Here's how the part is built. I have some questions about the finished solid (model axes, mm). A direction names the side the tool comes from. Give positions to 0.01 mm unless a question says otherwise; leave off trailing zeros. Loops run counter-clockwise (first coordinate to the right, second up) from the corner with the lowest first, then second, coordinate; pieces in that order, holes last. Notation, with made-up numbers: (-35.5, 56.5) - (-27.5, 56.5) arc R23 ccw to (-27.5, 90.5) - close; hole circle Ø5 at (83, 32). An arc over 180 degrees is marked (long way). Return JSON: item names as keys, results as strings. Group by question number.
(1) If we section it at D-D (z = 17.75): Please give me the cut outline in (x, y).
(2) If we mould it in two halves opening along X, with no side actions, what happens to faces 1 (the flat face through (-7.5, 26, 11)), 2 (the flat face through (41, 5, 14.45)), 3 (the flat face through (42.8, 5, 17))? For each: released by +X, released by -X, zero draft, split by the parting line, or undercut.
(3) If we section it at C-C (z = 10.5): Please give me the cut outline in (x, y).
(4) If we section it at B-B (y = 8): Please give me the cut outline in (x, z).
(5) On a 3-axis mill with a long thin cutter (end or side, diameter ignored), from which of +Z, -Z, +X, -X, +Y, -Y can I reach the whole of each face in a straight line? I mean faces 4 (the flat face through (28, 5, 2.5)), 5 (the flat face through (28, -90, 5)), 6 (the flat face through (-4, 26, 2.5)). Say none if no direction works.
(6) If we section it at A-A (x = 16.5): Please give me the cut outline in (y, z), then the cut area to 3 significant figures.
(7) For P1, Ø1, axis at y = -84, z = 10, coming from the +X side; P2, Ø0.7, axis at x = 7, z = 9, coming from the -Y side; P3, Ø8, axis at x = 25.5, y = 5, coming from the -Z side; P4, Ø2, axis at x = 30, z = 12.5, coming from the -Y side, each with a flat end and sliding along its axis, tell me the tip position at first contact or that it passes through.
(8) I need wall thicknesses on probe 1 along Y at (x, z) = (32, 6.25); probe 2 along X at (y, z) = (-111, 16); probe 3 along X at (y, z) = (8, 6). Which ranges of each line are inside material? Lowest first, please. Write a range as [from, to].
```python
from build123d import *

# Parameters (mm, degrees)
BOSS_EXTRUDE1_DEPTH      = 21.9
SKETCH2_W                = 4.7
SKETCH2_H                = 10
BOSS_EXTRUDE2_DEPTH      = 30
SKETCH3_W                = 5
SKETCH3_H                = 21.9
BOSS_EXTRUDE3_DEPTH      = 120
SKETCH4_W                = 3
SKETCH4_H                = 10
BOSS_EXTRUDE4_DEPTH      = 0.25
SKETCH5_W                = 3
SKETCH5_H                = 10
BOSS_EXTRUDE5_DEPTH      = 0.25
CORTE_EXTRUS_O1_DEPTH    = 10
ESBO_O3_W                = 21.9
ESBO_O3_H                = 7.5
RESSALTO_EXTRUS_O2_DEPTH = 10
ESBO_O4_W                = 7.5
ESBO_O4_H                = 16.9
CORTE_EXTRUS_O2_DEPTH    = 10
PADR_O_LINEAR1_COUNT     = 2
PADR_O_LINEAR1_PITCH     = 100


with BuildPart() as part:
    # Sketch1 → Boss-Extrude1 (new body)
    with BuildSketch(Plane.XY):
        Polygon((0, 0), (0, 30), (12.8, 30), (12.8, 0), (7.8, 0), (7.8, 10), (6, 10), (6, 0), align=None)
    extrude(amount=BOSS_EXTRUDE1_DEPTH)

    # Sketch2 → Boss-Extrude2 (add)
    with BuildSketch(Plane(origin=(12.8, 0, 0), x_dir=(0, 0, -1), z_dir=(1, 0, 0))):
        with Locations((-17.05, 5)):
            Rectangle(SKETCH2_W, SKETCH2_H)
        with Locations((-4.85, 5)):
            Rectangle(SKETCH2_W, SKETCH2_H)
    boss_extrude2 = extrude(amount=BOSS_EXTRUDE2_DEPTH)

    # Sketch3 → Boss-Extrude3 (add)
    with BuildSketch(Plane.XZ):
        with Locations((10.3, 10.95)):
            Rectangle(SKETCH3_W, SKETCH3_H)
    extrude(amount=BOSS_EXTRUDE3_DEPTH)

    # Sketch4 → Boss-Extrude4 (add)
    with BuildSketch(Plane(origin=(0, 0, 14.7), x_dir=(-1, 0, 0), z_dir=(0, 0, -1))):
        with Locations((-41.3, 5)):
            Rectangle(SKETCH4_W, SKETCH4_H)
    boss_extrude4 = extrude(amount=BOSS_EXTRUDE4_DEPTH)

    # Sketch5 → Boss-Extrude5 (add)
    with BuildSketch(Plane.XY.offset(7.2)):
        with Locations((41.3, 5)):
            Rectangle(SKETCH5_W, SKETCH5_H)
    boss_extrude5 = extrude(amount=BOSS_EXTRUDE5_DEPTH)

    # Esboço2 → Corte-extrusão1 (cut)
    with BuildSketch(Plane.XZ):
        with BuildLine():
            Line((6, 21.9), (6, 0))
            ThreePointArc((6, 0), (5.377380148, 10.95), (6, 21.9))
        make_face()
    extrude(amount=-CORTE_EXTRUS_O1_DEPTH, mode=Mode.SUBTRACT)

    # Esboço3 → Ressalto-extrusão2 (add)
    with BuildSketch(Plane.ZY):
        with Locations((10.95, 26.25)):
            Rectangle(ESBO_O3_W, ESBO_O3_H)
    extrude(amount=RESSALTO_EXTRUS_O2_DEPTH)

    # Esboço4 → Corte-extrusão2 (cut)
    with BuildSketch(Plane.XZ.offset(-22.5)):
        with Locations((-3.75, 10.95)):
            Rectangle(ESBO_O4_W, ESBO_O4_H)
    extrude(amount=-CORTE_EXTRUS_O2_DEPTH, mode=Mode.SUBTRACT)

    # Padrão linear1: Boss-Extrude2, Boss-Extrude4, Boss-Extrude5 ×2
    with Locations(*[(0, -i * PADR_O_LINEAR1_PITCH, 0) for i in range(1, PADR_O_LINEAR1_COUNT)]):
        add(boss_extrude2)
        add(boss_extrude4)
        add(boss_extrude5)


solid = part.part
```
Values:
{
 "1": {"outline": "(-10, 22.5) - (-7.5, 22.5) - (-7.5, 30) - (-10, 30) - close; (0, 0) - (5.62, 0) - (5.62, 10) - (7.8, 10) - (7.8, -120) - (12.8, -120) - (12.8, -100) - (42.8, -100) - (42.8, -90) - (12.8, -90) - (12.8, 0) - (42.8, 0) - (42.8, 10) - (12.8, 10) - (12.8, 30) - (0, 30) - close"},
 "2": {"face 1": "undercut", "face 2": "zero draft", "face 3": "released by +X"},
 "3": {"outline": "(-10, 22.5) - (-7.5, 22.5) - (-7.5, 30) - (-10, 30) - close; (0, 0) - (5.38, 0) - (5.38, 10) - (7.8, 10) - (7.8, -120) - (12.8, -120) - (12.8, 30) - (0, 30) - close"},
 "4": {"outline": "(0, 0) - (6, 0) arc R96.6 cw to (6, 21.9) - (0, 21.9) - close; (7.8, 0) - (12.8, 0) - (12.8, 2.5) - (42.8, 2.5) - (42.8, 7.45) - (39.8, 7.45) - (39.8, 7.2) - (12.8, 7.2) - (12.8, 14.7) - (39.8, 14.7) - (39.8, 14.45) - (42.8, 14.45) - (42.8, 19.4) - (12.8, 19.4) - (12.8, 21.9) - (7.8, 21.9) - close"},
 "5": {"face 4": "-Z, +X, +Y, -Y", "face 5": "+Z, -Z, +X", "face 6": "+Y, -Y"},
 "6": {"outline": "(-100, 2.5) - (-90, 2.5) - (-90, 7.2) - (-100, 7.2) - close; (-100, 14.7) - (-90, 14.7) - (-90, 19.4) - (-100, 19.4) - close; (0, 2.5) - (10, 2.5) - (10, 7.2) - (0, 7.2) - close; (0, 14.7) - (10, 14.7) - (10, 19.4) - (0, 19.4) - close", "area": "188 mm2"},
 "7": {"P1": "x = 12.8", "P2": "y = 10", "P3": "z = 2.5", "P4": "through"},
 "8": {"probe 1": "[-100, -90], [0, 10]", "probe 2": "[7.8, 12.8]", "probe 3": "[0, 5.5], [7.8, 42.8]"}
}
